The drawing under review shows one solid part. Ordinate dimensions are in mm from its lowest x, y, z. A direction names the side the tool comes from. Round coordinates to 2 decimals unless told otherwise and drop trailing zeros. Write each loop counter-clockwise with the first axis right and the second up, starting at its lowest first coordinate (ties: lowest second). Pieces come first, ordered by that corner, then holes. Notation, with made-up numbers: (20.5, -33.5) -> (76.5, -33.5) arc R19 ccw to (76.5, 1.5) -> close; hole circle Ø9 at (66.25, -14.5). An arc over 180 degrees is marked (long way). Answer in a Markdown table with one row per item. Add a question column.
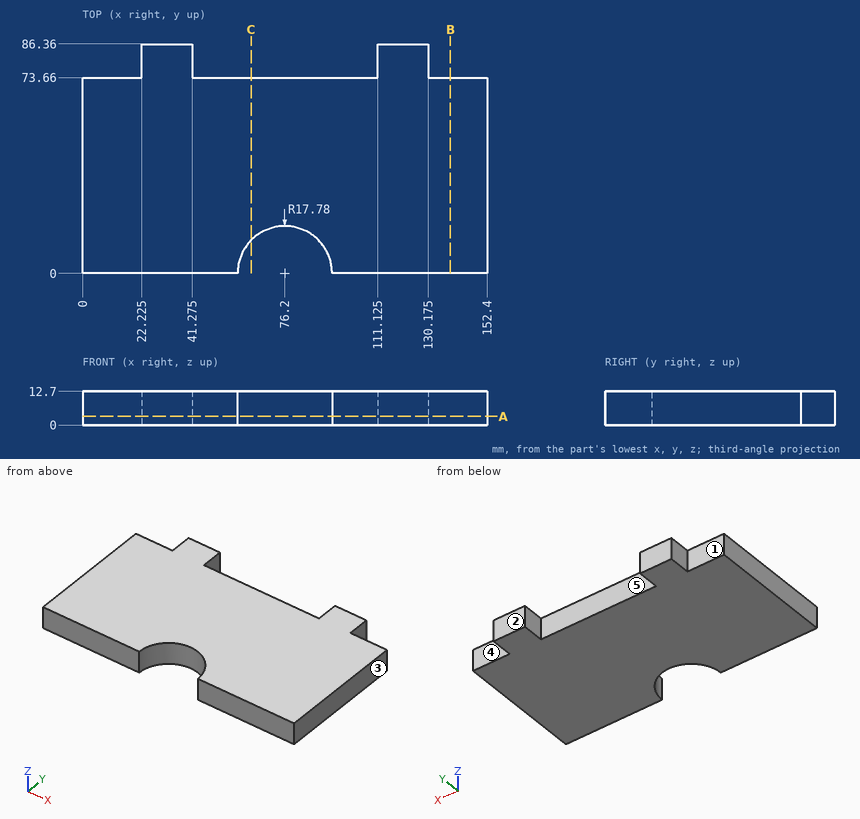
1. For L1, parallel to X at y = 74, z = 2 (3 decimals); L2, parallel to Y at x = 76.5, z = 0.75; L3, parallel to Y at x = 11, z = 11.5, list the stretches that pass through material, from the lowest coordinate up.
2. Add section A-A on z = 3.25. Write out the cut boundary in (x, y) (3 decimals).
3. Mouldability with a two-part tool opening along X and no side actions: class the marked faces 3, 4 and 5 as pulls with the +X half, pulls with the -X half, needs draft (parallel to the pull), parting line crosses it, or undercut.
4. Add section B-B on x = 138.5. Write out the cut boundary in (y, z), plus the area to 3 significant figures.
5. Tool access review of the marked faces 1 and 2: name each direction out of +Z, -Z, +X, -X, +Y, -Y from which nothing blocks a thin tool from reaching the whole face with its end or side.
6. Add section C-C on x = 63.5. Write out the cut boundary in (y, z).
7. Insertion check: pin 1 Ø5 at (x, z) = (100, 9) entering from -Y; pin 2 Ø4 at (y, z) = (80.5, 6.5) entering from -X (3 decimals); pin 3 Ø6.5 at (y, z) = (77, 7) entering from +X (3 decimals); pin 4 Ø3 at (x, z) = (88.5, 7) entering from -Y. Each pin has a flat end and moves straight along its axis. Give the tip position at first contact, or say it passes through.
Filled in:
| question | item | result |
|---|---|---|
| 1 | L1 | 22.225 to 41.275, 111.125 to 130.175 |
| 1 | L2 | 17.78 to 73.66 |
| 1 | L3 | 0 to 73.66 |
| 2 | outline | (0, 0) -> (58.42, 0) arc R17.78 cw to (93.98, 0) -> (152.4, 0) -> (152.4, 73.66) -> (130.175, 73.66) -> (130.175, 86.36) -> (111.125, 86.36) -> (111.125, 73.66) -> (41.275, 73.66) -> (41.275, 86.36) -> (22.225, 86.36) -> (22.225, 73.66) -> (0, 73.66) -> close |
| 3 | face 3 | pulls with the +X half |
| 3 | face 4 | needs draft |
| 3 | face 5 | undercut |
| 4 | outline | (0, 0) -> (73.66, 0) -> (73.66, 12.7) -> (0, 12.7) -> close |
| 4 | area | 935 mm² |
| 5 | face 1 | +Z, -Z, -X, +Y |
| 5 | face 2 | +Z, -Z, +X, -X, +Y |
| 6 | outline | (12.44, 0) -> (73.66, 0) -> (73.66, 12.7) -> (12.44, 12.7) -> close |
| 7 | pin 1 | y = 0 |
| 7 | pin 2 | x = 22.225 |
| 7 | pin 3 | x = 130.175 |
| 7 | pin 4 | y = 11.21 |
